Geometry: final body of the model. Coordinates: model frame, mm. A direction names the side the tool comes from. Give positions to 0.01 mm unless a question says otherwise; leave off trailing zeros. Order: outer loops, then holes, each group sorted by start corner. A loop starts at its lowest first (then second) coordinate and runs counter-clockwise, first axis right, second up. Notation, with made-up numbers: (66.5, -4.5) - (103.5, -4.5) arc R23 cw to (103.5, 25.5) - close; hole circle Ø3 at (67.5, 41.25). An arc over 180 degrees is marked (long way). Write item = value, one per line. Start each with the question number.
from build123d import *

# Parameters (mm, degrees)
SKETCH2_W           = 42.5
SKETCH2_H           = 25.8
BOSS_EXTRUDE1_DEPTH = 1.5
FILLET1_R           = 5
CHAMFER1_SIZE       = 0.7
BOSS_EXTRUDE2_DEPTH = 1.5
BOSS_EXTRUDE3_DEPTH = 1.7
FILLET2_R           = 0.6
SKETCH5_R           = 1.2
CUT_EXTRUDE1_DEPTH  = 26.039418923


with BuildPart() as part:
    # Sketch2 → Boss-Extrude1 (new body)
    with BuildSketch(Plane(origin=(0, 0, 0), x_dir=(1, 0, 0), z_dir=(0, 1, 0))):
        Rectangle(SKETCH2_W, SKETCH2_H)
    extrude(amount=BOSS_EXTRUDE1_DEPTH)

    # Fillet1
    fillet1_edges = [part.edges().sort_by_distance(p)[0] for p in [
        (21.25, 0.75, -12.9),
        (21.25, 0.75, 12.9),
        (-21.25, 0.75, 12.9),
        (-21.25, 0.75, -12.9),
    ]]
    fillet(fillet1_edges, radius=FILLET1_R)

    # Chamfer1
    chamfer1_edges = [part.edges().sort_by_distance(p)[0] for p in [
        (21.25, 1.5, 0),
        (0, 1.5, 12.9),
        (0, 1.5, -12.9),
        (-21.25, 1.5, 0),
        (-19.785533906, 1.5, 11.435533906),
        (-19.785533906, 1.5, -11.435533906),
        (19.785533906, 1.5, -11.435533906),
        (19.785533906, 1.5, 11.435533906),
    ]]
    chamfer(chamfer1_edges, length=CHAMFER1_SIZE)

    # Sketch3 → Boss-Extrude2 (add)
    with BuildSketch(Plane(origin=(0, 0, 0), x_dir=(1, 0, 0), z_dir=(0, 1, 0))):
        with BuildLine():
            Line((17.75, 1.3), (-17.75, 1.3))
            ThreePointArc((-17.75, 1.3), (-19.05, 0), (-17.75, -1.3))
            Line((-17.75, -1.3), (17.75, -1.3))
            ThreePointArc((17.75, -1.3), (19.05, 0), (17.75, 1.3))
        make_face()
        with BuildLine():
            Line((12.5, 10.7), (-12.5, 10.7))
            ThreePointArc((-12.5, 10.7), (-13.8, 9.4), (-12.5, 8.1))
            Line((-12.5, 8.1), (12.5, 8.1))
            ThreePointArc((12.5, 8.1), (13.8, 9.4), (12.5, 10.7))
        make_face()
        with BuildLine():
            Line((12.5, -8.1), (-12.5, -8.1))
            ThreePointArc((-12.5, -8.1), (-13.8, -9.4), (-12.5, -10.7))
            Line((-12.5, -10.7), (12.5, -10.7))
            ThreePointArc((12.5, -10.7), (13.8, -9.4), (12.5, -8.1))
        make_face()
    extrude(amount=-BOSS_EXTRUDE2_DEPTH)

    # Sketch4 → Boss-Extrude3 (add)
    with BuildSketch(Plane.XZ.offset(1.5)):
        with BuildLine():
            Line((17.75, 1.3), (-17.75, 1.3))
            ThreePointArc((-17.75, 1.3), (-19.05, 0), (-17.75, -1.3))
            Line((-17.75, -1.3), (17.75, -1.3))
            ThreePointArc((17.75, -1.3), (19.05, 0), (17.75, 1.3))
        make_face()
    extrude(amount=BOSS_EXTRUDE3_DEPTH)

    # Fillet2
    fillet2_edges = [part.edges().sort_by_distance(p)[0] for p in [
        (19.05, -3.2, 0),
        (0, -3.2, -1.3),
        (-19.05, -3.2, 0),
        (0, -3.2, 1.3),
    ]]
    fillet(fillet2_edges, radius=FILLET2_R)

    # Sketch5 → Cut-Extrude1 (cut, through all)
    with BuildSketch(Plane.XZ.offset(1.5)):
        with Locations(Location((-12.5, 9.4, 0), (0, 0, 270))):
            Circle(SKETCH5_R)
        with Locations(Location((12.5, 9.4, 0), (0, 0, 270))):
            Circle(SKETCH5_R)
        with Locations(Location((12.5, -9.4, 0), (0, 0, 270))):
            Circle(SKETCH5_R)
        with Locations(Location((-12.5, -9.4, 0), (0, 0, 270))):
            Circle(SKETCH5_R)
    extrude(amount=-CUT_EXTRUDE1_DEPTH, mode=Mode.SUBTRACT)


solid = part.part
Q1. Set-up query: faces 5 (the cylindrical face through (-19.05, -1.28, 0.03)), 6 (the flat face through (0, -1, 10.7)), 7 (the flat face through (0, -1.5, -9)), 8 (the flat face through (0, -1, -1.3)). Return all of +Z, -Z, +X, -X, +Y, -Y with unobstructed straight access to the full face (end or side cutting, diameter ignored); none if empty.
Q2. Section B-B, the plane x = -3.5. Return the cut outline in (y, z), then the cut area to 3 significant figures.
Q3. Pull-direction query (Z, two-part tool) for faces 1 (the cylindrical face through (-12.14, -0.021, 8.255)), 2 (the flat face through (0, -1, -10.7)), 3 (the conical face through (19.34, 1.38, 11.06)), 4 (the cylindrical face through (-11.689, -0.021, -8.516)); classes: +Z half, -Z half, draft (parallel to the pull), parting line (faces both ways), or undercut.
Q4. Material intervals for line 1 along Z through (x, y) = (9.5, -0.6); line 2 along X through (y, z) = (0.4, 9.4); line 3 along Y through (x, z) = (6, -1.5), sorted ascending. Write a range as from..to.
Q5. Section C-C, the plane z = 4.75. Return the cut outline in (x, y).
Q6. Contact query for flat-ended pins moving along their axis: pin 1 (1.2 mm diameter, centred on x = 4.5, y = -1, fed in from -Z); pin 2 (1.6 mm diameter, centred on x = -6, y = -0.5, fed in from -Z); pin 3 (1.2 mm diameter, centred on x = -3.5, y = -1, fed in from +Z); pin 4 (3 mm diameter, centred on x = 5.5, z = -9.5, fed in from -Y). Output: stop coordinate, or through.
Q7. Section D-D, the plane y = -2.1. Return the cut outline in (x, z), then the cut area to 3 significant figures.
Q8. Section A-A, the plane x = 13. Return the cut outline in (y, z), then the cut area to 3 significant figures.
The answers:
q1.face_5 = -X, -Y
q1.face_6 = +Z, +X, -X, -Y
q1.face_7 = -Z, +X, -X, -Y
q1.face_8 = +X, -X, -Y
q2.outline = (-3.2, -0.7) arc R0.6 ccw to (-2.6, -1.3) - (0, -1.3) - (0, -8.1) - (-1.5, -8.1) - (-1.5, -10.7) - (0, -10.7) - (0, -12.9) - (0.8, -12.9) - (1.5, -12.2) - (1.5, 12.2) - (0.8, 12.9) - (0, 12.9) - (0, 10.7) - (-1.5, 10.7) - (-1.5, 8.1) - (0, 8.1) - (0, 1.3) - (-2.6, 1.3) arc R0.6 ccw to (-3.2, 0.7) - close
q2.area = 54.2 mm²
q3.face_1 = undercut
q3.face_2 = -Z half
q3.face_3 = +Z half
q3.face_4 = undercut
q4.line_1 = -10.7..-8.1, -1.3..1.3, 8.1..10.7
q4.line_2 = -21.02..-13.7, -11.3..11.3, 13.7..21.02
q4.line_3 = 0..1.5
q5.outline = (-21.25, 0) - (21.25, 0) - (21.25, 0.8) - (20.55, 1.5) - (-20.55, 1.5) - (-21.25, 0.8) - close
q6.pin_1 = -10.7
q6.pin_2 = -12.9
q6.pin_3 = 10.7
q6.pin_4 = -1.5
q7.outline = (-17.75, -1.3) - (17.75, -1.3) arc R1.3 ccw to (17.75, 1.3) - (-17.75, 1.3) arc R1.3 ccw to start
q7.area = 97.6 mm²
q8.outline = (-3.2, -0.7) arc R0.6 ccw to (-2.6, -1.3) - (0, -1.3) - (0, -8.2) - (-1.5, -8.2) - (-1.5, -8.31) - (1.5, -8.31) - (1.5, 8.31) - (-1.5, 8.31) - (-1.5, 8.2) - (0, 8.2) - (0, 1.3) - (-2.6, 1.3) arc R0.6 ccw to (-3.2, 0.7) - close; (-1.5, -10.6) - (0, -10.6) - (0, -12.9) - (0.8, -12.9) - (1.5, -12.2) - (1.5, -10.49) - (-1.5, -10.49) - close; (-1.5, 10.49) - (1.5, 10.49) - (1.5, 12.2) - (0.8, 12.9) - (0, 12.9) - (0, 10.6) - (-1.5, 10.6) - close
q8.area = 40.5 mm²
